from build123d import *

# Parameters (mm, degrees)
SKETCH_R        = 6.25
SKETCH_R_2      = 4
PAD_DEPTH       = 8
PAD001_DEPTH    = 3
FILLET_R        = 1.5
FILLET001_R     = 1
SKETCH002_W     = 2
SKETCH002_H     = 10
SKETCH002_W_2   = 10
SKETCH002_H_2   = 2
PAD002_DEPTH    = 2
CHAMFER_SIZE    = 1.99
SKETCH003_R     = 6.26
SKETCH003_R_2   = 5.58
POCKET_DEPTH    = 3
SKETCH004_W     = 1
SKETCH004_H     = 14
POCKET001_DEPTH = 20
CHAMFER001_SIZE = 0.6
CHAMFER002_SIZE = 1


with BuildPart() as part:
    # Sketch → Pad (new body)
    with BuildSketch(Plane.XY):
        with Locations((15, 15)):
            Circle(SKETCH_R)
        with Locations((15, 15)):
            Circle(SKETCH_R_2, mode=Mode.SUBTRACT)
    extrude(amount=PAD_DEPTH)

    # Sketch001 (on Face3 of Pad) → Pad001 (join)
    with BuildSketch(Plane(origin=(0, 0, 0), x_dir=(1, 0, 0), z_dir=(0, 0, -1))):
        with BuildLine():
            Line((0, -28.504743), (0, 0))
            Line((0, 0), (28.504743, 0))
            ThreePointArc((30.002374, -1.584264), (29.594788, -0.469562), (28.504743, 0))
            ThreePointArc((1.584264, -30.002374), (21.216341, -21.216341), (30.002374, -1.584264))
            ThreePointArc((0, -28.504743), (0.469562, -29.594788), (1.584264, -30.002374))
        make_face()
    extrude(amount=PAD001_DEPTH)

    # Fillet
    fillet_edges = [part.edges().sort_by_distance(p)[0] for p in [
        (0, 0, -1.5),
    ]]
    fillet(fillet_edges, radius=FILLET_R)

    # Fillet001
    fillet001_edges = [part.edges().sort_by_distance(p)[0] for p in [
        (0, 15.002371, -3),
        (0.43934, 0.43934, -3),
        (0.469562, 29.594788, -3),
        (15.002371, 0, -3),
        (21.216341, 21.216341, -3),
        (29.594788, 0.469562, -3),
    ]]
    fillet(fillet001_edges, radius=FILLET001_R)

    # Sketch002 (on Face4 of Fillet001) → Pad002 (join)
    with BuildSketch(Plane.XY):
        with Locations((6, 15)):
            Rectangle(SKETCH002_W, SKETCH002_H)
        with Locations((15, 6)):
            Rectangle(SKETCH002_W_2, SKETCH002_H_2)
    extrude(amount=PAD002_DEPTH)

    # Chamfer
    chamfer_edges = [part.edges().sort_by_distance(p)[0] for p in [
        (15, 5, 0),
        (5, 15, 0),
    ]]
    chamfer(chamfer_edges, length=CHAMFER_SIZE)

    # Sketch003 → Pocket (cut)
    with BuildSketch(Plane.XY):
        with Locations((15, 15)):
            Circle(SKETCH003_R)
        with Locations((15, 15)):
            Circle(SKETCH003_R_2, mode=Mode.SUBTRACT)
    extrude(amount=POCKET_DEPTH, mode=Mode.SUBTRACT)

    # Sketch004 (on Face1 of Pocket) → Pocket001 (cut)
    with BuildSketch(Plane.XY):
        with Locations((15, 15)):
            Rectangle(SKETCH004_W, SKETCH004_H)
    extrude(amount=POCKET001_DEPTH, mode=Mode.SUBTRACT)

    # Chamfer001
    chamfer001_edges = [part.edges().sort_by_distance(p)[0] for p in [
        (19.118641, 11.235269, 0),
        (9.42, 15, 0),
        (9.42, 15, 3),
        (19.118641, 11.235269, 3),
        (8.75, 15, 8),
        (19.592793, 10.761044, 8),
    ]]
    chamfer(chamfer001_edges, length=CHAMFER001_SIZE)

    # Chamfer002
    chamfer002_edges = [part.edges().sort_by_distance(p)[0] for p in [
        (11, 15, 0),
        (18, 17.645751, 0),
    ]]
    chamfer(chamfer002_edges, length=CHAMFER002_SIZE)


solid = part.part
Geometry check sheet. Reference: the model listing, model coordinates, mm. A direction names the side the tool comes from. Give positions to 0.01 mm unless a question says otherwise; leave off trailing zeros. Order: outer loops, then holes, each group sorted by start corner. A loop starts at its lowest first (then second) coordinate and runs counter-clockwise, first axis right, second up. Notation, with made-up numbers: (59, 50.5) - (65, 50.5) arc R20 cw to (65, 62.5) - close; hole circle Ø7 at (32.25, 16.25). An arc over 180 degrees is marked (long way). Answer as a JSON object with one key per item and string values.
(1) Cross-section at B-B (z = -1). Record the cut outline in (x, y), then the cut area to 3 significant figures.
Report:
{"outline": "(0, 1.5) arc R1.5 ccw to (1.5, 0) - (28.5, 0) arc R1.5 ccw to (30, 1.58) arc R30.16 ccw to (1.58, 30) arc R1.5 ccw to (0, 28.5) - close", "area": "706 mm^2"}
(2) Tool access check on faces 1 (the cylindrical face through (8.75, 15.13, 5.17)), 2 (the flat face through (14.5, 10, 4)), 3 (the conical face through (11.8, 15.1, 0.2)). Record the directions out of +Z, -Z, +X, -X, +Y, -Y that give a thin tool (end or side, any length) a straight path to the whole face; none if there is none.
Report:
{"face 1": "+Z, -X", "face 2": "+Z, +Y", "face 3": "+Z"}
(3) Material ranges on line 1 (X direction, y = 15.5, z = 1.5); line 2 (Z direction, x = 21, y = 10.5); line 3 (X direction, y = 19, z = 1), recorded low to high.
Report:
{"line 1": "4.51 to 7, 9.44 to 11.03, 18.97 to 20.56", "line 2": "-3 to 0", "line 3": "4.01 to 7, 11.11 to 14.5, 15.5 to 18.89"}
(4) Depth check by flat-ended pin: pin 1 Ø3.5 at (y, z) = (20, 3.5) entering from +X; pin 2 Ø1.6 at (y, z) = (10, 5) entering from -X; pin 3 Ø3.5 at (y, z) = (9.5, 3) entering from +X; pin 4 Ø6 at (x, z) = (27, 2.5) entering from -Y. Enter the tip coordinate at first touch or a pass-through.
Report:
{"pin 1": "x = 20.34", "pin 2": "x = 10.37", "pin 3": "x = 20", "pin 4": "y = 0"}
(5) Draft check along Y on faces 4 (the cylindrical face through (20.58, 14.88, 1.49)), 5 (the flat face through (5, 10, 1)), 6 (the flat face through (0, 15, -1)), 7 (the conical face through (20.82, 15.12, 7.83)). Enter one of: released by +Y, released by -Y, zero draft, split by the parting line, or undercut.
Report:
{"face 4": "undercut", "face 5": "released by -Y", "face 6": "zero draft", "face 7": "split by the parting line"}
(6) Cross-section at A-A (z = 7). Record the cut outline in (x, y).
Report:
{"outline": "(14.5, 8.77) - (14.5, 11.03) arc R4 cw to (14.5, 18.97) - (14.5, 21.23) arc R6.25 ccw to start; (15.5, 8.77) arc R6.25 ccw to (15.5, 21.23) - (15.5, 18.97) arc R4 cw to (15.5, 11.03) - close"}
